Here's how the part is built. I have some questions about the finished solid (model axes, mm). A direction names the side the tool comes from. Coordinates: 2 decimals unless noted, no trailing zeros. Write each loop counter-clockwise with the first axis right and the second up, starting at its lowest first coordinate (ties: lowest second). Pieces come first, ordered by that corner, then holes.
Item 1: I want a section at C-C (z = 7.25). Please give me the cut outline in (x, y) (3 decimals), and give its area (3 significant figures).
Item 2: I'm going to push flat-ended pins straight in: P1, Ø1.5, axis at y = 3, z = 12, coming from the -X side; P2, Ø5.5, axis at x = 0, y = 0, coming from the -Z side; P3, Ø5, axis at y = -5, z = 15, coming from the +X side; P4, Ø1.5, axis at y = -4.5, z = 3, coming from the +X side. Where does each tip first touch, or does it pass through?
Item 3: If we mould it in two halves opening along X, with no side actions, what happens to faces 1 (the face through (5.172, -3.042, 8.381)), 2 (the face through (0, -6, 8)), 3 (the face through (1.344, 3.639, 6.551))? For each: pulls with the +X half, pulls with the -X half, needs draft (parallel to the pull), parting line crosses it, or undercut.
Item 4: I want a section at B-B (x = 0). Please give me the cut outline in (y, z) (3 decimals), and give its area (3 significant figures).
Item 5: I want a section at A-A (z = 9.5). Please give me the cut outline in (x, y) (3 decimals), and give its area (3 significant figures).
Item 6: Please list where these lines run through material, in increasing order: line 1 (Y direction, x = 0, z = 13.5); line 2 (X direction, y = -1.5, z = 2.25); line 3 (Y direction, x = -1.25, z = 11).
Item 7: For faces 4 (the face through (-0.439, -1.977, 4.93)), 5 (the face through (0, 6, 10)), 6 (the face through (1.48, 3.64, 3.08)), which set-ups out of +Z, -Z, +X, -X, +Y, -Y let a thin tool reach every point of the face, with its end or its side?
Item 8: I want a section at D-D (y = 3). Please give me the cut outline in (x, z) (3 decimals), and give its area (3 significant figures).
from build123d import *

# Parameters (mm, degrees)
F_01_17_MM_COMMERCIAL_DRIVE_HEX_DEPTH  = 17
F_02_START                             = -0.1
S02_SHAFT_SEAT_R                       = 2.025
F_02_SHAFT_SEAT_DEPTH                  = 10.1
F_03_START                             = 9.99
S03_OUTBOARD_M4_THREAD_ENVELOPE_R      = 1.65
F_03_OUTBOARD_M4_THREAD_ENVELOPE_DEPTH = 7.11
S04_RADIAL_M3_SET_SCREW_1_R            = 1.515
F_04_RADIAL_M3_SET_SCREW_1_DEPTH       = 7
S05_RADIAL_M3_SET_SCREW_2_R            = 1.515
F_05_RADIAL_M3_SET_SCREW_2_DEPTH       = 7


with BuildPart() as part:
    # S01 - 17 mm commercial drive hex → 01 - 17 mm commercial drive hex (new body)
    with BuildSketch(Plane.XY):
        Polygon((6.92820323, 0), (3.464101615, 6), (-3.464101615, 6), (-6.92820323, 0), (-3.464101615, -6), (3.464101615, -6), align=None)
    extrude(amount=F_01_17_MM_COMMERCIAL_DRIVE_HEX_DEPTH)

    # S02 - Shaft seat → 02 - Shaft seat (cut)
    with BuildSketch(Plane.XY.offset(F_02_START)):
        Circle(S02_SHAFT_SEAT_R)
    extrude(amount=F_02_SHAFT_SEAT_DEPTH, mode=Mode.SUBTRACT)

    # S03 - Outboard M4 thread envelope → 03 - Outboard M4 thread envelope (cut)
    with BuildSketch(Plane.XY.offset(F_03_START)):
        Circle(S03_OUTBOARD_M4_THREAD_ENVELOPE_R)
    extrude(amount=F_03_OUTBOARD_M4_THREAD_ENVELOPE_DEPTH, mode=Mode.SUBTRACT)

    # S04 - Radial M3 set screw 1 → 04 - Radial M3 set screw 1 (cut)
    with BuildSketch(Plane(origin=(0, 0, 0), x_dir=(1, 0, 0), z_dir=(0, 1, 0))):
        with Locations(Location((0, -2.75, 0), (0, 0, 90))):
            Circle(S04_RADIAL_M3_SET_SCREW_1_R)
    extrude(amount=F_04_RADIAL_M3_SET_SCREW_1_DEPTH, mode=Mode.SUBTRACT)

    # S05 - Radial M3 set screw 2 → 05 - Radial M3 set screw 2 (cut)
    with BuildSketch(Plane(origin=(0, 0, 0), x_dir=(1, 0, 0), z_dir=(0, 1, 0))):
        with Locations(Location((0, -7.25, 0), (0, 0, 90))):
            Circle(S05_RADIAL_M3_SET_SCREW_2_R)
    extrude(amount=F_05_RADIAL_M3_SET_SCREW_2_DEPTH, mode=Mode.SUBTRACT)


solid = part.part
Answer:
1. outline: (-6.928, 0) - (-3.464, -6) - (3.464, -6) - (6.928, 0) - (3.464, 6) - (1.515, 6) - (1.515, 1.344) arc R2.025 cw (long way) to (-1.515, 1.344) - (-1.515, 6) - (-3.464, 6) - close
1. area: 99.1 mm2
2. P1: stops at x = -5.63
2. P2: stops at z = 0
2. P3: stops at x = 5.48
2. P4: stops at x = 4.76
3. face 1: pulls with the +X half
3. face 2: needs draft
3. face 3: undercut
4. outline: (-6, 0) - (-2.025, 0) - (-2.025, 10) - (-1.65, 10) - (-1.65, 17) - (-6, 17) - close; (1.65, 10) - (2.025, 10) - (2.025, 8.765) - (6, 8.765) - (6, 17) - (1.65, 17) - close; (2.025, 0) - (6, 0) - (6, 1.235) - (2.025, 1.235) - close; (2.025, 4.265) - (6, 4.265) - (6, 5.735) - (2.025, 5.735) - close
4. area: 116 mm2
5. outline: (-6.928, 0) - (-3.464, -6) - (3.464, -6) - (6.928, 0) - (3.464, 6) - (-3.464, 6) - close; hole circle Ø4.05 at (0, 0)
5. area: 112 mm2
6. line 1: y = -6 to -1.65, 1.65 to 6
6. line 2: x = -6.06 to -1.36, 1.36 to 6.06
6. line 3: y = -6 to -1.08, 1.08 to 6
7. face 4: -Z
7. face 5: +Z, -Z, +X, -X, +Y
7. face 6: +Y
8. outline: (-5.196, 0) - (5.196, 0) - (5.196, 17) - (-5.196, 17) - close; hole circle Ø3.03 at (0, 2.75); hole circle Ø3.03 at (0, 7.25)
8. area: 162 mm2
